Input: part model. Units: mm. Frame: model coordinates. Give positions to 0.01 mm unless a question says otherwise; leave off trailing zeros. Loops run counter-clockwise (first coordinate to the right, second up) from the corner with the lowest first, then second, coordinate; pieces in that order, holes last. Notation, with made-up numbers: M -17,10.5 L 23,10.5 A16 ccw 23,18.5 Z; hole C 30,-22.5 d6. An arc over 180 degrees is marked long. Use CSV: the item, a comma, the result in double quotes. Start each with the question number.
Q1. Pin query (flat end, axial travel): pin 1 (1.5 mm diameter, centred on y = 1, z = 56.5, fed in from -X); pin 2 (1.5 mm diameter, centred on x = 661.5, y = 2, fed in from -Z); pin 3 (2.5 mm diameter, centred on x = 666.13, z = 43.46, fed in from -Y); pin 4 (0.9 mm diameter, centred on x = 666, y = 1.5, fed in from +Z). Return the tip coordinate at first contact, or that it passes through.
Q2. Section C-C, the plane z = 21. Output: boundary loops of the cut face in (x, y), plus the area to 3 significant figures.
Q3. Material intervals for line 1 along X through (y, z) = (1, -7.5); line 2 along Z through (x, y) = (665.5, 2.1); line 3 along X through (y, z) = (2.45, 59), sorted ascending.
Q4. Pull-direction query (X, two-part tool) for faces 1 (the cylindrical face through (646, 2, -13)), 2 (the cylindrical face through (656.652, 1.479, 51.644)), 3 (the flat face through (673, 1, 3)), 4 (the flat face through (662.4, 1.52, 56.01)); classes: released by +X, released by -X, zero draft, split by the parting line, or undercut.
Q5. Section B-B, the plane z = 9.5. Output: boundary loops of the cut face in (x, y), plus the area to 3 significant figures.
Q6. Section A-A, the plane z = -7.5. Output: boundary loops of the cut face in (x, y).
Q7. Section D-D, the plane y = 1.45. State how many separate pieces and enclosed holes the cut face has, plus the area to 3 significant figures.
from build123d import *

# Parameters (mm, degrees)
SKETCH_1_R          = 1.45
EXTRUDE_1_DEPTH     = 3
FILLET_1_R          = 5
CUT_EXTRUDE_1_DEPTH = 685.034246793
FILLET_2_R          = 1.5


with BuildPart() as part:
    # 草图1 → 凸台-拉伸1 (new body)
    with BuildSketch(Plane(origin=(0, 0, 0), x_dir=(1, 0, 0), z_dir=(0, 1, 0))):
        Polygon((650.079202112, -57.331500941), (648.989953088, -72.291899885), (678.910750976, -74.470397934), (680, -59.50999899), (680, -3), (665, -3), (665, 15), (645, 15), (645, 0), (651.894617153, -32.397502701), align=None)
        with Locations(Location((660, 7.5, 0), (0, 0, 270))):
            Circle(SKETCH_1_R, mode=Mode.SUBTRACT)
        with Locations(Location((650, 7.5, 0), (0, 0, 270))):
            Circle(SKETCH_1_R, mode=Mode.SUBTRACT)
        with Locations(Location((654.521377248, -65.174783421, 0), (0, 0, 270))):
            Circle(SKETCH_1_R, mode=Mode.SUBTRACT)
        with Locations(Location((674.46857584, -66.627115454, 0), (0, 0, 270))):
            Circle(SKETCH_1_R, mode=Mode.SUBTRACT)
        with Locations(Location((666.12885008, -43.460351022, 0), (0, 0, 270))):
            Circle(SKETCH_1_R, mode=Mode.SUBTRACT)
        with Locations(Location((668.307348129, -13.539553134, 0), (0, 0, 270))):
            Circle(SKETCH_1_R, mode=Mode.SUBTRACT)
    extrude(amount=EXTRUDE_1_DEPTH)

    # 圆角1
    fillet_1_edges = [part.edges().sort_by_distance(p)[0] for p in [
        (678.910750976, 1.5, 74.470397934),
        (648.989953088, 1.5, 72.291899885),
        (651.894617153, 1.5, 32.397502701),
        (645, 1.5, 0),
        (645, 1.5, -15),
        (665, 1.5, -15),
        (665, 1.5, 3),
        (680, 1.5, 3),
    ]]
    fillet(fillet_1_edges, radius=FILLET_1_R)

    # 草图2 → 切除-拉伸1 (cut, through all)
    with BuildSketch(Plane(origin=(0, 3, 0), x_dir=(1, 0, 0), z_dir=(0, 1, 0))):
        Polygon((649.367123648, 3.5), (655.178416972, -23.807011685), (662, 3.5), align=None)
        Polygon((660.867017044, -17.539553134), (675, -17.539553134), (675, -39.460351022), (655.390967722, -39.460351022), align=None)
        Polygon((659.946903123, -47.460351022), (671.444064599, -47.460351022), (665.695483861, -67.49232755), align=None)
        Polygon((655.390967722, -42.460351022), (655.390967722, -61.174783421), (660.76145253, -61.174783421), align=None)
        Polygon((676, -42.460351022), (670.212739147, -62.627115454), (676, -62.627115454), align=None)
    extrude(amount=-CUT_EXTRUDE_1_DEPTH, mode=Mode.SUBTRACT)

    # 圆角2
    fillet_2_edges = [part.edges().sort_by_distance(p)[0] for p in [
        (655.390967722, 1.5, 39.460351022),
        (660.867017044, 1.5, 17.539553134),
        (675, 1.5, 17.539553134),
        (675, 1.5, 39.460351022),
        (665.695483861, 1.5, 67.49232755),
        (659.946903123, 1.5, 47.460351022),
        (671.444064599, 1.5, 47.460351022),
        (676, 1.5, 42.460351022),
        (676, 1.5, 62.627115454),
        (670.212739147, 1.5, 62.627115454),
        (655.390967722, 1.5, 42.460351022),
        (660.76145253, 1.5, 61.174783421),
        (655.390967722, 1.5, 61.174783421),
        (649.367123648, 1.5, -3.5),
        (662, 1.5, -3.5),
        (655.178416972, 1.5, 23.807011685),
        (680, 1.5, 59.50999899),
    ]]
    fillet(fillet_2_edges, radius=FILLET_2_R)


solid = part.part
A:
1,pin 1,"x = 650.09"
1,pin 2,"z = -14.94"
1,pin 3,"through"
1,pin 4,"z = 73.56"
2,outline,"M 649.47,0 L 660,0 L 660,3 L 649.47,3 Z; M 675,0 L 680,0 L 680,3 L 675,3 Z"
2,area,"46.6 mm^2"
3,line 1,"645 to 648.55, 651.45 to 658.55, 661.45 to 665"
3,line 2,"0.18 to 17.54, 39.46 to 42.15, 44.77 to 47.46, 63.54 to 73.49"
3,line 3,"649.96 to 655.39, 660.14 to 663.26, 668.13 to 671.25, 676 to 680"
4,face 1,"released by -X"
4,face 2,"undercut"
4,face 3,"zero draft"
4,face 4,"undercut"
5,outline,"M 647.02,0 L 652.13,0 L 652.13,3 L 647.02,3 Z; M 658.75,0 L 680,0 L 680,3 L 658.75,3 Z"
5,area,"79.1 mm^2"
6,outline,"M 645,0 L 648.55,0 L 648.55,3 L 645,3 Z; M 651.45,0 L 658.55,0 L 658.55,3 L 651.45,3 Z; M 661.45,0 L 665,0 L 665,3 L 661.45,3 Z"
7,separate pieces,"1"
7,enclosed holes,"11"
7,area,"1,700 mm^2"
